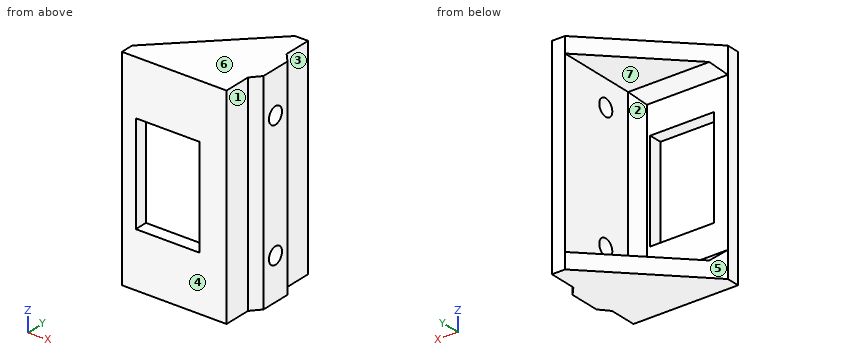
```python
from build123d import *

# Parameters (mm, degrees)
PAD_DEPTH       = 40
PAD001_DEPTH    = 3
PAD002_DEPTH    = 3
PAD003_DEPTH    = 40
SKETCH004_W     = 12.2
SKETCH004_H     = 19
POCKET_DEPTH    = 2.5
SKETCH005_R     = 1.6
POCKET001_DEPTH = 4.06
CHAMFER_SIZE    = 2


with BuildPart() as part:
    # Sketch → Pad (new body)
    with BuildSketch(Plane.XY):
        Polygon((0, 0), (0, 20), (-2.5, 20), (-2.5, 2.5), (-20, 2.5), (-20, 0), align=None)
    extrude(amount=PAD_DEPTH)

    # Sketch001 (on Face8 of Pad) → Pad001 (join)
    with BuildSketch(Plane.XY.offset(40)):
        Polygon((-2.5, 20), (-20, 2.5), (-2.5, 2.5), align=None)
    extrude(amount=-PAD001_DEPTH)

    # Sketch002 (on Face4 of Pad001) → Pad002 (join)
    with BuildSketch(Plane(origin=(0, 0, 0), x_dir=(1, 0, 0), z_dir=(0, 0, -1))):
        Polygon((-20, -2.5), (-2.5, -20), (-2.5, -2.5), align=None)
    extrude(amount=-PAD002_DEPTH)

    # Sketch003 (on Face4 of Pad002) → Pad003 (join)
    with BuildSketch(Plane(origin=(0, 0, 0), x_dir=(1, 0, 0), z_dir=(0, 0, -1))):
        Polygon((0, -5.26), (0, -14.74), (1.56, -12.94), (1.56, -7.06), align=None)
    extrude(amount=-PAD003_DEPTH)

    # Sketch004 (on Face18 of Pad003) → Pocket (cut)
    with BuildSketch(Plane(origin=(0, 2.5, 0), x_dir=(-1, 0, 0), z_dir=(0, 1, 0))):
        with Locations((11.25, 20)):
            Rectangle(SKETCH004_W, SKETCH004_H)
    extrude(amount=-POCKET_DEPTH, mode=Mode.SUBTRACT)

    # Sketch005 (on Face12 of Pocket) → Pocket001 (cut)
    with BuildSketch(Plane.YZ.offset(1.56)):
        with Locations((10, 32)):
            Circle(SKETCH005_R)
        with Locations((10, 8)):
            Circle(SKETCH005_R)
    extrude(amount=-POCKET001_DEPTH, mode=Mode.SUBTRACT)

    # Chamfer
    chamfer_edges = [part.edges().sort_by_distance(p)[0] for p in [
        (-11.25, 2.5, 3),
        (-2.5, 2.5, 20),
        (-11.25, 2.5, 37),
    ]]
    chamfer(chamfer_edges, length=CHAMFER_SIZE)


solid = part.part
```
The model under review builds one solid part; all positions refer to its coordinate system, in mm. Face numbers are marked on the shaded views. A direction names the side the tool comes from. Coordinates: 2 decimals unless noted, no trailing zeros. Write each loop counter-clockwise with the first axis right and the second up, starting at its lowest first coordinate (ties: lowest second). Pieces come first, ordered by that corner, then holes. Notation, with made-up numbers: (55, -37.5) -> (92, -37.5) arc R19 cw to (92, -28.5) -> close; hole circle Ø6 at (38.25, 34.25). An arc over 180 degrees is marked (long way). One line per item, written item: value. Start each with the question number.
Q1. Add section B-B, the plane z = 8. Give the boundary of the cut face in (x, y), then the cut area to 3 significant figures.
Q2. Add section A-A, the plane x = -16. Give the boundary of the cut face in (y, z), then the cut area to 3 significant figures.
Q3. Clearance check with flat-ended pins moving along their axes: P1, Ø1.6, axis at y = 1.5, z = 26, coming from the +X side; P2, Ø3.5, axis at y = 10, z = 32, coming from the -X side; P3, Ø8, axis at x = -14.5, z = 15, coming from the +Y side. State where each tip first meets the part, or that it passes through.
Q4. To check wall thickness, follow probe 1 along Z at (x, y) = (0.1, 10); probe 2 along Z at (x, y) = (-11.25, 6); probe 3 along X at (y, z) = (18.5, 22.5). State the ranges of each line that lie inside material, in increasing order.
Q5. Add section C-C, the plane y = 10. Give the boundary of the cut face in (x, z), then the cut area to 3 significant figures.
Q6. The part is to be moulded in two halves that separate along Z. For the marked faces 5, 6 and 7, say which applies: +Z half, -Z half, draft (parallel to the pull), parting line (faces both ways), or undercut.
Q7. Add section D-D, the plane y = 17.25. Give the boundary of the cut face in (x, z), then the cut area to 4 significant figures.
Q8. For the marked faces 1, 2, 3 and 4, list the 3-axis set-ups (+Z, -Z, +X, -X, +Y, -Y) from which the entire face can be reached by the end or side of a thin tool; tool diameter is ignored.
Response:
1. outline: (-20, 0) -> (0, 0) -> (0, 5.26) -> (1.56, 7.06) -> (1.56, 8.4) -> (-2.5, 8.4) -> (-2.5, 4.5) -> (-4.5, 2.5) -> (-20, 2.5) -> close; (-2.5, 11.6) -> (1.56, 11.6) -> (1.56, 12.94) -> (0, 14.74) -> (0, 20) -> (-2.5, 20) -> close
1. area: 94.7 mm²
2. outline: (0, 0) -> (6.5, 0) -> (6.5, 3) -> (4.5, 3) -> (2.5, 5) -> (2.5, 10.5) -> (0, 10.5) -> close; (0, 29.5) -> (2.5, 29.5) -> (2.5, 35) -> (4.5, 37) -> (6.5, 37) -> (6.5, 40) -> (0, 40) -> close
2. area: 80.5 mm²
3. P1: x = 0
3. P2: x = -2.5
3. P3: y = 2.5
4. probe 1: 0 to 6.4, 9.6 to 30.4, 33.6 to 40
4. probe 2: 0 to 3, 37 to 40
4. probe 3: -2.5 to 0
5. outline: (-12.5, 0) -> (1.56, 0) -> (1.56, 6.4) -> (-2.5, 6.4) -> (-2.5, 3) -> (-12.5, 3) -> close; (-12.5, 37) -> (-2.5, 37) -> (-2.5, 33.6) -> (1.56, 33.6) -> (1.56, 40) -> (-12.5, 40) -> close; (-2.5, 9.6) -> (1.56, 9.6) -> (1.56, 30.4) -> (-2.5, 30.4) -> close
5. area: 196 mm²
6. face 5: draft
6. face 6: +Z half
6. face 7: undercut
7. outline: (-5.25, 0) -> (0, 0) -> (0, 40) -> (-5.25, 40) -> (-5.25, 37) -> (-2.5, 37) -> (-2.5, 3) -> (-5.25, 3) -> close
7. area: 116.5 mm²
8. face 1: +Z, -Z, +X, -Y
8. face 2: -X, +Y
8. face 3: +Z, -Z, +X, +Y
8. face 4: +Z, -Z, +X, -X, -Y
